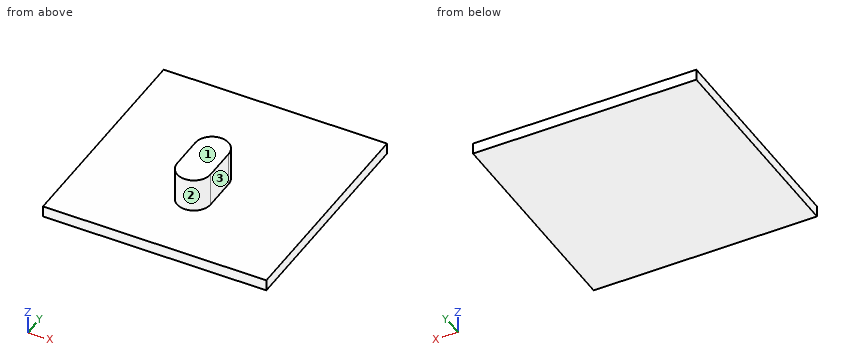
```python
from build123d import *

# Parameters (mm, degrees)
SKETCH_1_W      = 40
SKETCH_1_H      = 40
EXTRUDE_1_DEPTH = 2
SKETCH_1_3_R    = 3
EXTRUDE_2_DEPTH = 8


with BuildPart() as part:
    # Sketch 1 → Extrude 1 (new body)
    with BuildSketch(Plane.XY):
        Rectangle(SKETCH_1_W, SKETCH_1_H)
        with BuildLine():
            ThreePointArc((3, -7), (0, -10), (-3, -7))
            Line((-3, -7), (-3, -1))
            ThreePointArc((-3, -1), (0, 2), (3, -1))
            Line((3, -1), (3, -7))
        make_face(mode=Mode.SUBTRACT)
    extrude(amount=EXTRUDE_1_DEPTH)

    # Sketch 1_3 → Extrude 2 (add)
    with BuildSketch(Plane.XY):
        with Locations((0, -1)):
            Circle(SKETCH_1_3_R)
        with BuildLine():
            Line((-3, -1), (-3, -7))
            ThreePointArc((-3, -7), (-2.121320344, -4.878679656), (0, -4))
            ThreePointArc((0, -4), (-2.121320344, -3.121320344), (-3, -1))
        make_face()
        with BuildLine():
            ThreePointArc((0, -4), (2.121320344, -4.878679656), (3, -7))
            Line((3, -7), (3, -1))
            ThreePointArc((3, -1), (2.121320344, -3.121320344), (0, -4))
        make_face()
        with Locations((0, -7)):
            Circle(SKETCH_1_3_R)
    extrude(amount=EXTRUDE_2_DEPTH)


solid = part.part
```
Read the model definition and answer for the solid it produces. Units are mm, in the model's axes. Face numbers are marked on the shaded views. A direction names the side the tool comes from. Give positions to 0.01 mm unless a question says otherwise; leave off trailing zeros. Write each loop counter-clockwise with the first axis right and the second up, starting at its lowest first coordinate (ties: lowest second). Pieces come first, ordered by that corner, then holes. Notation, with made-up numbers: (-36, 35.5) - (-30, 35.5) arc R25 ccw to (-30, 62.5) - close; hole circle Ø3 at (-28, 33). An arc over 180 degrees is marked (long way). Write item = value, one per line. Start each with the question number.
Item 1: Find section C-C (z = 4.5). Give the vertices of the cut face in (x, y), then the cut area to 3 significant figures.
Item 2: A tool of negligible diameter and unlimited length cuts with its end or side. For the marked faces 1, 2 and 3, from which of +Z, -Z, +X, -X, +Y, -Y can it reach the whole face along a straight path? Write none if from no direction.
Item 3: Find section A-A (x = 0). Give the vertices of the cut face in (y, z).
Item 4: Find section D-D (x = 14). Give the vertices of the cut face in (y, z), then the cut area to 3 significant figures.
Item 5: Find the intervals of material crossed by probe 1 along Z at (x, y) = (-10, -9); probe 2 along X at (y, z) = (-4, 4); probe 3 along X at (y, z) = (1, 4.25), in increasing order. Write a range as [from, to].
Item 6: Find section B-B (y = -7.5). Give the vertices of the cut face in (x, z).
Item 7: Each of these flat-tipped pins is pushed along its axis until it touches: P1, Ø3, axis at y = -5, z = 4, coming from the +X side; P2, Ø2, axis at x = -5, y = -8.5, coming from the +Z side. Where does it stop, or does it pass through?
Response:
q1.outline = (-3, -7) arc R3 ccw to (3, -7) - (3, -1) arc R3 ccw to (-3, -1) - close
q1.area = 64.3 mm²
q2.face_1 = +Z, +X, -X, +Y, -Y
q2.face_2 = +Z, -Y
q2.face_3 = +Z, +X, +Y, -Y
q3.outline = (-20, 0) - (20, 0) - (20, 2) - (2, 2) - (2, 8) - (-10, 8) - (-10, 2) - (-20, 2) - close
q4.outline = (-20, 0) - (20, 0) - (20, 2) - (-20, 2) - close
q4.area = 80.0 mm²
q5.probe_1 = [0, 2]
q5.probe_2 = [-3, 3]
q5.probe_3 = [-2.24, 2.24]
q6.outline = (-20, 0) - (20, 0) - (20, 2) - (2.96, 2) - (2.96, 8) - (-2.96, 8) - (-2.96, 2) - (-20, 2) - close
q7.P1 = 3
q7.P2 = 2
